Autodesk Inventor part; units mm, degrees
ref_plane "YZ Plane" through (0, 0, 0) normal (1, 0, 0) x (0, 1, 0)
ref_plane "XZ Plane" through (0, 0, 0) normal (0, 1, 0) x (-1, 0, 0)
ref_plane "XY Plane" through (0, 0, 0) normal (0, 0, 1) x (1, 0, 0)
sketch "Sketch1" plane through (0, 0, 0) normal (0, 1, 0) x (-1, 0, 0)
  line L0 (97, 285) -> (-97, 285)
  line L1 (-97, 285) -> (-97, -285)
  line L2 (-97, -285) -> (97, -285)
  line L3 (97, -285) -> (97, 285)
  point P0 (0, 0)
  dimension "d0" = 194
  dimension "d1" = 570
  dimension "d2" = 97
  dimension "d3" = 285
extrude "Plate1" add sketch "Sketch1" along normal blind 3.048
sketch "Sketch3" plane through (100.048, 6.096, -285) normal (1, 0, 0) x (0, 1, 0)
  line L0 (0, 570) -> (0, 0)
  line L1 (0, 0) -> (3.904, 0)
  line L2 (3.904, 0) -> (3.904, 570)
  line L3 (3.904, 570) -> (0, 570)
edge flange "Flange1" height 10 angle 90 thickness 3.048 bend radius 3.048 thickness toward (1, 0, 0) relief tear relief width 3.048 relief depth 1.524 edges at (97, 3.048, 0) wall of the first edge with corners at (100.048, 6.096, 285) (100.048, 6.096, -285) (100.048, 10, -285) (100.048, 10, 285)
bend "Bend1"
corner "Corner1"
equation "\"d4\" = Thickness"
equation "\"d5\" = BendReliefWidth"
equation "\"d6\" = BendReliefDepth"
equation "\"d7\" = MinimumRemnant"
equation "\"d8\" = TransitionRadius"
equation "\"d11\" = BendRadius"
equation "\"d12\" = CornerReliefSize"
equation "\"d13\" = GapSize"
equation "\"d14\" = JacobiRadiusSize"
equation "\"BendRadius\" = Thickness"
equation "\"BendReliefWidth\" = Thickness"
equation "\"BendReliefDepth\" = 0.5 * Thickness"
equation "\"CornerReliefSize\" = 4 * Thickness"
equation "\"MinimumRemnant\" = 2 * Thickness"
equation "\"TransitionRadius\" = BendRadius"
equation "\"JacobiRadiusSize\" = BendRadius"
equation "\"GapSize\" = Thickness"
properties part number "CO-1-01-controlsSeperator"
Input: part model. Units: mm. Frame: model coordinates. A direction names the side the tool comes from. Coordinates: 2 decimals unless noted, no trailing zeros. Loops run counter-clockwise (first coordinate to the right, second up) from the corner with the lowest first, then second, coordinate; pieces in that order, holes last. Notation, with made-up numbers: M 36.25,3.25 L 51.25,3.25 A9 ccw 51.25,17.25 Z; hole C -1,-23.75 d7. An arc over 180 degrees is marked long. Use a Markdown table: item, result. Add a question column.
1) Set-up query: faces 1 (the flat face through (1, 0, 4)), 2 (the flat face through (1, 3.048, 4)). Return all of +Z, -Z, +X, -X, +Y, -Y with unobstructed straight access to the full face (end or side cutting, diameter ignored); none if empty.
2) Section B-B, the plane x = 8. Return the cut outline in (y, z), plus the area to 3 significant figures.
3) Section A-A, the plane z = 85.5. Return the cut outline in (x, y).
4) Line query: L1, parallel to Y at x = 46.5, z = 153; L2, parallel to X at y = 8.5, z = 240; L3, parallel to X at y = 1.25, z = 189. Output: solid intervals per line, ascending. Write a range as from..to.
5) Pin query (flat end, axial travel): P1, Ø2, axis at x = 72.5, z = 88.5, coming from the -Y side; P2, Ø4.5, axis at y = 8, z = -71.5, coming from the -X side. Return the tip coordinate at first contact, or that it passes through.
Answer below:
| question | item | result |
|---|---|---|
| 1 | face 1 | +Z, -Z, +X, -X, -Y |
| 1 | face 2 | +Z, -Z, -X, +Y |
| 2 | outline | M 0,-285 L 3.05,-285 L 3.05,285 L 0,285 Z |
| 2 | area | 1,740 mm2 |
| 3 | outline | M -97,0 L 97,0 A6.1 ccw 103.1,6.1 L 103.1,10 L 100.05,10 L 100.05,6.1 A3.05 cw 97,3.05 L -97,3.05 Z |
| 4 | L1 | 0..3.05 |
| 4 | L2 | 100.05..103.1 |
| 4 | L3 | -97..100.7 |
| 5 | P1 | y = 0 |
| 5 | P2 | x = 100.03 |
